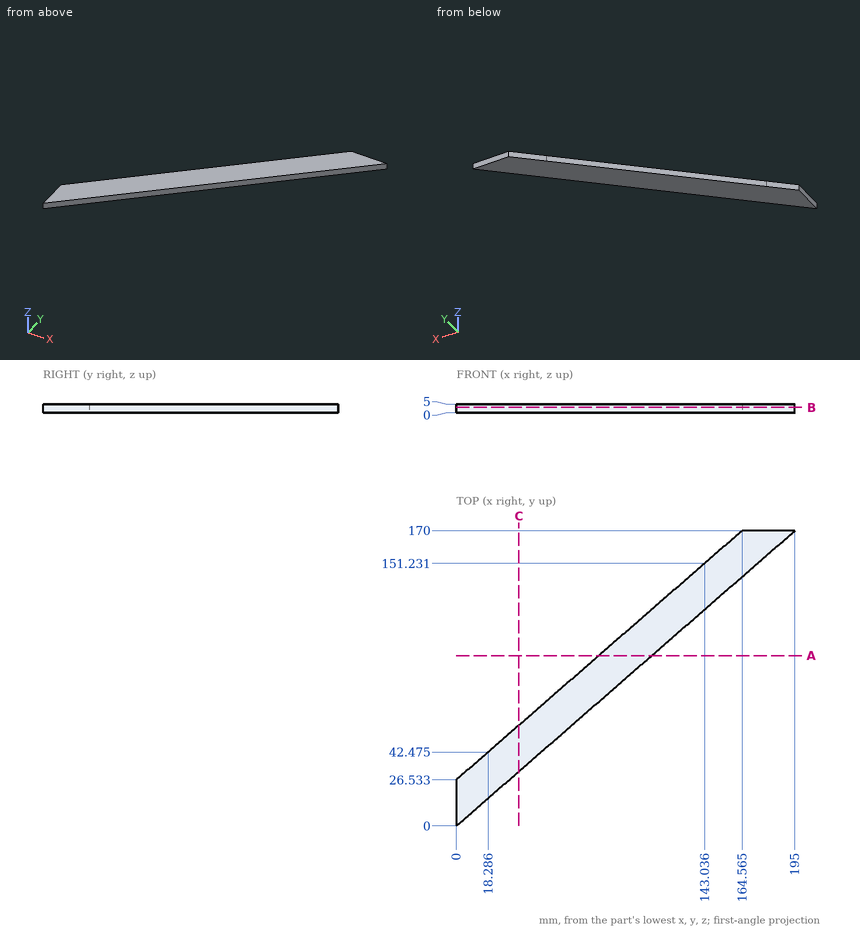
Geometry: see drawing. Coordinates: mm, zero at the bounding-box minimum. Round coordinates to 2 decimals unless told otherwise and drop trailing zeros. Write each loop counter-clockwise with the first axis right and the second up, starting at its lowest first coordinate (ties: lowest second). Pieces come first, ordered by that corner, then holes. Notation, with made-up numbers: (-27.5, 23) -> (17.5, 23) arc R12 ccw to (17.5, 41) -> close; hole circle Ø4 at (85.25, 76). An arc over 180 degrees is marked (long way). Answer as CSV lines item,"result".
1. Contact query for flat-ended pins moving along their axis: P1, Ø2, axis at x = 106, z = 3, coming from the +Y side (1 decimal); P2, Ø1.5, axis at x = 99, z = 2, coming from the -Y side (1 decimal); P3, Ø1.5, axis at y = 124, z = 4, coming from the -X side. Output: stop coordinate, or through.
Geometry says:
P1,"stops at y = 119.8"
P2,"stops at y = 85.7"
P3,"stops at x = 110.94"
2. Section B-B (z = 3.1). Return the cut outline in (x, y) (1 decimal).
Geometry says:
outline,"(0, 0) -> (195, 170) -> (164.6, 170) -> (18.3, 42.5) -> (0, 26.5) -> close"
3. Section C-C (x = 36). Return the cut outline in (y, z) (1 decimal).
Geometry says:
outline,"(31.4, 0) -> (57.9, 0) -> (57.9, 5) -> (31.4, 5) -> close"
4. Section A-A (y = 98). Return the cut outline in (x, z).
Geometry says:
outline,"(81.98, 0) -> (112.41, 0) -> (112.41, 5) -> (81.98, 5) -> close"
5. Ray query, L1, parallel to X at y = 60, z = 4.6 (1 decimal); L2, parallel to X at y = 48, z = 2.85 (1 decimal); L3, parallel to Y at x = 152, z = 1.9 (1 decimal). Return the intervals inside material, ascending. Write a range as [from, to].
Geometry says:
L1,"x = [38.4, 68.8]"
L2,"x = [24.6, 55.1]"
L3,"y = [132.5, 159]"
